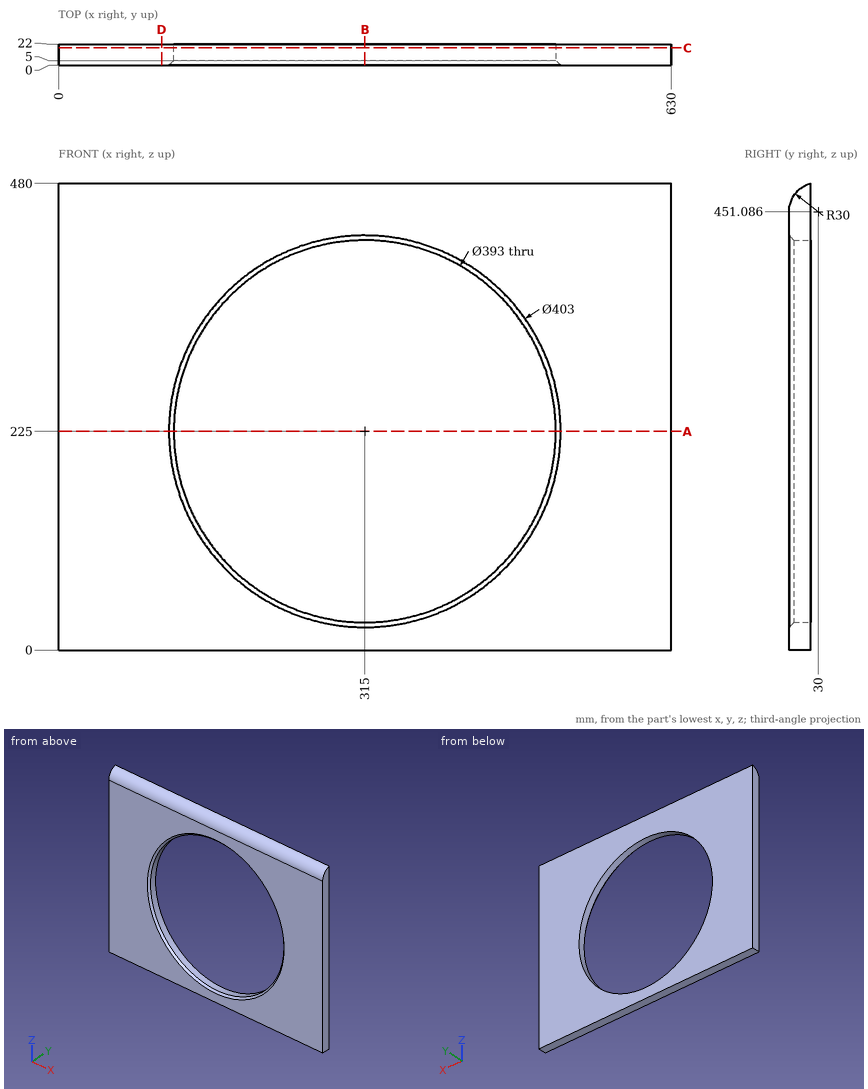
Input: dimensioned drawing with shaded views. Units: mm. Origin: part minimum x, y, z. Give positions to 0.01 mm unless a question says otherwise; leave off trailing zeros. Write each loop counter-clockwise with the first axis right and the second up, starting at its lowest first coordinate (ties: lowest second). Pieces come first, ordered by that corner, then holes. Notation, with made-up numbers: M 68.25,68 L 126.25,68 A18 cw 126.25,86 Z; hole C -25.5,-18.75 d5. An arc over 180 degrees is marked long. Return JSON: item names as keys, results as strings. Group by question number.
1) Cut plane B-B, the plane x = 315. Output: boundary loops of the cut face in (y, z), plus the area to 3 significant figures.
2) Cut plane C-C, the plane y = 18. Output: boundary loops of the cut face in (x, z).
3) Pin query (flat end, axial travel): P1, Ø6, axis at x = 212.5, y = 9, coming from the +Z side; P2, Ø4, axis at x = 332, y = 16, coming from the +Z side; P3, Ø3, axis at x = 208, y = 9, coming from the +Z side (1 decimal). Return the tip coordinate at first contact, or that it passes through.
4) Material intervals for line 1 along X through (y, z) = (5.5, 125.5) (1 decimal); line 2 along X through (y, z) = (13, 271.5); line 3 along Z through (x, y) = (414, 13.75) (1 decimal), sorted ascending. Write a range as [from, to].
5) Cut plane D-D, the plane x = 106. Output: boundary loops of the cut face in (y, z), plus the area to 3 significant figures.
6) Cut plane A-A, the plane z = 225. Output: boundary loops of the cut face in (x, y), plus the area to 3 significant figures.
Recorded:
{
 "1": {"outline": "M 0,0 L 22,0 L 22,28.5 L 5,28.5 L 0,23.5 Z; M 0,426.5 L 5,421.5 L 22,421.5 L 22,480 A30 ccw 0,451.09 Z", "area": "1,720 mm²"},
 "2": {"outline": "M 0,0 L 630,0 L 630,478.58 L 0,478.58 Z; hole C 315,225 d393"},
 "3": {"P1": "stops at z = 475.09", "P2": "stops at z = 478.58", "P3": "stops at z = 473.9"},
 "4": {"line 1": "x = [0, 145.6], [484.4, 630]", "line 2": "x = [0, 124.08], [505.92, 630]", "line 3": "z = [0, 55.3], [394.7, 476.3]"},
 "5": {"outline": "M 0,0 L 22,0 L 22,480 A30 ccw 0,451.09 Z", "area": "10,400 mm²"},
 "6": {"outline": "M 0,0 L 113.5,0 L 118.5,5 L 118.5,22 L 0,22 Z; M 511.5,5 L 516.5,0 L 630,0 L 630,22 L 511.5,22 Z", "area": "5,190 mm²"}
}
